```python
from build123d import *

# Parameters (mm, degrees)
SKETCH1_W                = 105.85
SKETCH1_H                = 66.84
BOSS_EXTRUDE1_DEPTH      = 3.175
SKETCH2_W                = 8.1
SKETCH2_H                = 3.225
SKETCH2_W_2              = 3.225
SKETCH2_H_2              = 8.1
CUT_EXTRUDE1_DEPTH       = 63.674018939
SKETCH3_W                = 8
SKETCH3_H                = 8
BOSS_EXTRUDE2_DEPTH      = 3.175
M3_CLEARANCE_HOLE1_D     = 3.2
M3_CLEARANCE_HOLE1_DEPTH = 12
M3_CLEARANCE_HOLE1_TIP   = 0.96137699
CUT_EXTRUDE2_DEPTH       = 70.56171828
FILLET1_R                = 1
FILLET2_R                = 3


with BuildPart() as part:
    # Sketch1 → Boss-Extrude1 (new body)
    with BuildSketch(Plane(origin=(0, 0, 0), x_dir=(1, 0, 0), z_dir=(0, 1, 0))):
        Rectangle(SKETCH1_W, SKETCH1_H)
    extrude(amount=BOSS_EXTRUDE1_DEPTH)

    # Sketch2 → Cut-Extrude1 (cut, through all)
    with BuildSketch(Plane(origin=(0, 3.175, 0), x_dir=(1, 0, 0), z_dir=(0, 1, 0))):
        with Locations((-35, 31.8075)):
            Rectangle(SKETCH2_W, SKETCH2_H)
        with Locations((35, 31.8075)):
            Rectangle(SKETCH2_W, SKETCH2_H)
        with Locations((35, -31.8075)):
            Rectangle(SKETCH2_W, SKETCH2_H)
        with Locations((-35, -31.8075)):
            Rectangle(SKETCH2_W, SKETCH2_H)
        with Locations((-51.3125, -15)):
            Rectangle(SKETCH2_W_2, SKETCH2_H_2)
        with Locations((-51.3125, 15)):
            Rectangle(SKETCH2_W_2, SKETCH2_H_2)
    extrude(amount=-CUT_EXTRUDE1_DEPTH, mode=Mode.SUBTRACT)

    # Sketch3 → Boss-Extrude2 (add)
    with BuildSketch(Plane(origin=(0, 3.175, 0), x_dir=(1, 0, 0), z_dir=(0, 1, 0))):
        with Locations((56.925, 29.42)):
            Rectangle(SKETCH3_W, SKETCH3_H)
        with Locations((56.925, -29.42)):
            Rectangle(SKETCH3_W, SKETCH3_H)
    extrude(amount=-BOSS_EXTRUDE2_DEPTH)

    # M3 Clearance Hole1
    with Locations(Plane(origin=(0, 3.175, 0), x_dir=(1, 0, 0), z_dir=(0, 1, 0))):
        with Locations((56.925, 29.42), (56.925, -29.42), (-25.245, 15), (-25.245, -15)):
            Hole(M3_CLEARANCE_HOLE1_D / 2, depth=M3_CLEARANCE_HOLE1_DEPTH)
            with Locations((0, 0, -(M3_CLEARANCE_HOLE1_DEPTH + M3_CLEARANCE_HOLE1_TIP / 2))):  # 118° drill point
                Cone(0, M3_CLEARANCE_HOLE1_D / 2, M3_CLEARANCE_HOLE1_TIP, mode=Mode.SUBTRACT)

    # Sketch10 → Cut-Extrude2 (cut, through all)
    with BuildSketch(Plane(origin=(0, 3.175, 0), x_dir=(1, 0, 0), z_dir=(0, 1, 0))):
        Polygon((-34.126976843, 23.767082591), (34.126976843, 23.767082591), (0, 3.489615661), align=None)
        Polygon((-40, 20.27746693), (-5.873023157, 0), (-40, -20.27746693), align=None)
        Polygon((-34.126976843, -23.767082591), (0, -3.489615661), (34.126976843, -23.767082591), align=None)
        Polygon((40, -20.27746693), (40, 20.27746693), (5.873023157, 0), align=None)
    extrude(amount=-CUT_EXTRUDE2_DEPTH, mode=Mode.SUBTRACT)

    # Fillet1
    fillet1_edges = [part.edges().sort_by_distance(p)[0] for p in [
        (60.925, 1.5875, -33.42),
        (60.925, 1.5875, 33.42),
        (-52.925, 1.5875, 33.42),
        (-52.925, 1.5875, -33.42),
    ]]
    fillet(fillet1_edges, radius=FILLET1_R)

    # Fillet2
    fillet2_edges = [part.edges().sort_by_distance(p)[0] for p in [
        (34.126976843, 1.5875, 23.767082591),
        (-34.126976843, 1.5875, 23.767082591),
        (0, 1.5875, 3.489615661),
        (-40, 1.5875, 20.27746693),
        (-40, 1.5875, -20.27746693),
        (-5.873023157, 1.5875, 0),
        (40, 1.5875, 20.27746693),
        (5.873023157, 1.5875, 0),
        (40, 1.5875, -20.27746693),
        (0, 1.5875, -3.489615661),
        (-34.126976843, 1.5875, -23.767082591),
        (34.126976843, 1.5875, -23.767082591),
    ]]
    fillet(fillet2_edges, radius=FILLET2_R)


solid = part.part
```
Design review of the part built by this model. Coordinates are the model's own, in mm. A direction names the side the tool comes from. Give positions to 0.01 mm unless a question says otherwise; leave off trailing zeros. Order: outer loops, then holes, each group sorted by start corner. A loop starts at its lowest first (then second) coordinate and runs counter-clockwise, first axis right, second up. Notation, with made-up numbers: (-22.75, 72) -> (5.25, 72) arc R20 cw to (5.25, 109) -> close; hole circle Ø2 at (63.5, 54). An arc over 180 degrees is marked (long way). Write item = value, one per line. Start each with the question number.
(1) We need section B-B on x = 6.5. Write out the cut boundary in (y, z) (3 decimals), plus the area to 3 significant figures.
(2) For faces 4 (the face through (-30.95, 2, -32)), 5 (the face through (22.7, 1.6, 10)), 6 (the face through (35, 2, 30.195)), list the 3-axis set-ups (+Z, -Z, +X, -X, +Y, -Y) from which the entire face can be reached by the end or side of a thin tool; tool diameter is ignored.
(3) To check wall thickness, follow line 1 along X through (y, z) = (1.6, 15) (3 decimals); line 2 along X through (y, z) = (1.65, -8) (3 decimals); line 3 along Z through (x, y) = (25, 0.9). State the ranges of each line that lie inside material, in increasing order.
(4) Mouldability with a two-part tool opening along Z and no side actions: class faces 1 (the face through (49, 2, -33.42)), 2 (the face through (0, 2, 33.42)), 3 (the face through (0.02, 1.57, 3.98)) as +Z half, -Z half, draft (parallel to the pull), parting line (faces both ways), or undercut.
(5) We need section C-C on y = 2.55. State how many separate pieces and enclosed holes the cut face has, plus the area to 3 significant figures.
(6) For pin 1 (1.6 mm diameter, centred on y = 2, z = 4.5, fed in from +X) (3 decimals); pin 2 (1.6 mm diameter, centred on x = 34, y = 1.5, fed in from -Z) (3 decimals), all flat-tipped, find the tip position at first contact; note any pin that passes through.
(7) We need section A-A on z = -9.5. Write out the cut boundary in (x, y) (3 decimals), plus the area to 3 significant figures.
Numbers:
q1.outline = (0, -33.42) -> (3.175, -33.42) -> (3.175, -23.767) -> (0, -23.767) -> close; (0, -7.352) -> (3.175, -7.352) -> (3.175, 7.352) -> (0, 7.352) -> close; (0, 23.767) -> (3.175, 23.767) -> (3.175, 33.42) -> (0, 33.42) -> close
q1.area = 108 mm^2
q2.face_4 = -Z, +Y, -Y
q2.face_5 = +Y, -Y
q2.face_6 = +Z, +Y, -Y
q3.line_1 = -49.7 to -40, -31.118 to -26.845, -23.645 to -19.372, 19.372 to 31.118, 40 to 52.925
q3.line_2 = -52.925 to -40, -19.337 to -7.591, 7.591 to 19.337, 40 to 52.925
q3.line_3 = -33.42 to -23.17, -18.36 to -11.36, 11.36 to 18.36, 23.17 to 33.42
q4.face_1 = -Z half
q4.face_2 = +Z half
q4.face_3 = undercut
q5.separate_pieces = 1
q5.enclosed_holes = 8
q5.area = 4,370 mm^2
q6.pin_1 = 52.925
q6.pin_2 = -30.195
q7.outline = (-52.925, 0) -> (-40, 0) -> (-40, 3.175) -> (-52.925, 3.175) -> close; (-21.862, 0) -> (-10.115, 0) -> (-10.115, 3.175) -> (-21.862, 3.175) -> close; (10.115, 0) -> (21.862, 0) -> (21.862, 3.175) -> (10.115, 3.175) -> close; (40, 0) -> (52.925, 0) -> (52.925, 3.175) -> (40, 3.175) -> close
q7.area = 157 mm^2
